```python
from build123d import *

# Parameters (mm, degrees)
F0_W     = 35
F0_H     = 50
F1_DEPTH = 40.208638
F2_R     = 10
F3_R     = 9.604884
F4_DEPTH = 72.155587


with BuildPart() as f1:
    # F0 (on Top) → F1 (new body)
    with BuildSketch(Plane.XY):
        with Locations((17.5, 25)):
            Rectangle(F0_W, F0_H)
    extrude(amount=F1_DEPTH)

    # F2
    f2_edges = [f1.edges().sort_by_distance(p)[0] for p in [
        (17.5, 0, 40.208638),
        (17.5, 50, 40.208638),
    ]]
    fillet(f2_edges, radius=F2_R)

    # F3 (on face) → F4 (cut)
    with BuildSketch(Plane.XY.offset(40.208638)):
        with Locations((17.5, 25)):
            Circle(F3_R)
    extrude(amount=-F4_DEPTH, mode=Mode.SUBTRACT)

    # F5: F1 across face


with BuildPart() as f1_1:
    add(f1.part)
    add(f1.part.mirror(Plane(origin=(35, 25, 19.714479), x_dir=(0, 1, 0), z_dir=(1, 0, 0))))


solid = f1_1.part
```
Model file for the job. Use its own axes, mm. Give positions to 0.01 mm unless a question says otherwise; leave off trailing zeros. Order: outer loops, then holes, each group sorted by start corner. A loop starts at its lowest first (then second) coordinate and runs counter-clockwise, first axis right, second up.
1) Saw through at A-A, the plane x = 52.5. Write the cut outline in (y, z).
2) Saw through at C-C, the plane z = 14.5. Write the cut outline in (x, y), then the cut area to 3 significant figures.
3) Saw through at B-B, the plane y = 25. Write the cut outline in (x, z).
4) Pin check, flat tip, straight feed: pin 1 (17.5 mm diameter, centred on x = 52.5, y = 25, fed in from +Z). Stop position of the tip, or through.
5) Mould opens along X. For faces 1 (the cylindrical face through (60, 19, 20)), 2 (the flat face through (0, 25, 20)), 3 (the cylindrical face through (10, 19, 20)), 4 (the flat face through (35, 50, 15)) say: +X half, -X half, draft (parallel to the pull), parting line (faces both ways), or undercut.
6) Wall check: probe 1 along X at (y, z) = (25.5, 33.5); probe 2 along X at (y, z) = (28.5, 35.5); probe 3 along Y at (x, z) = (52.5, 20). Give the ranges that are in metal, low to high.
7) Saw through at D-D, the plane x = 37.5. Write the cut outline in (y, z), then the cut area to 3 significant figures.
Computed:
1. outline: (0, 0) - (15.4, 0) - (15.4, 40.21) - (10, 40.21) arc R10 ccw to (0, 30.21) - close; (34.6, 0) - (50, 0) - (50, 30.21) arc R10 ccw to (40, 40.21) - (34.6, 40.21) - close
2. outline: (0, 0) - (70, 0) - (70, 50) - (0, 50) - close; hole circle Ø19.21 at (17.5, 25); hole circle Ø19.21 at (52.5, 25)
2. area: 2,920 mm2
3. outline: (0, 0) - (7.9, 0) - (7.9, 40.21) - (0, 40.21) - close; (27.1, 0) - (42.9, 0) - (42.9, 40.21) - (27.1, 40.21) - close; (62.1, 0) - (70, 0) - (70, 40.21) - (62.1, 40.21) - close
4. pin 1: passes through
5. face 1: undercut
5. face 2: -X half
5. face 3: undercut
5. face 4: draft
6. probe 1: x = 0 to 7.91, 27.09 to 42.91, 62.09 to 70
6. probe 2: x = 0 to 8.56, 26.44 to 43.56, 61.44 to 70
6. probe 3: y = 0 to 15.4, 34.6 to 50
7. outline: (0, 0) - (50, 0) - (50, 30.21) arc R10 ccw to (40, 40.21) - (10, 40.21) arc R10 ccw to (0, 30.21) - close
7. area: 1,970 mm2
